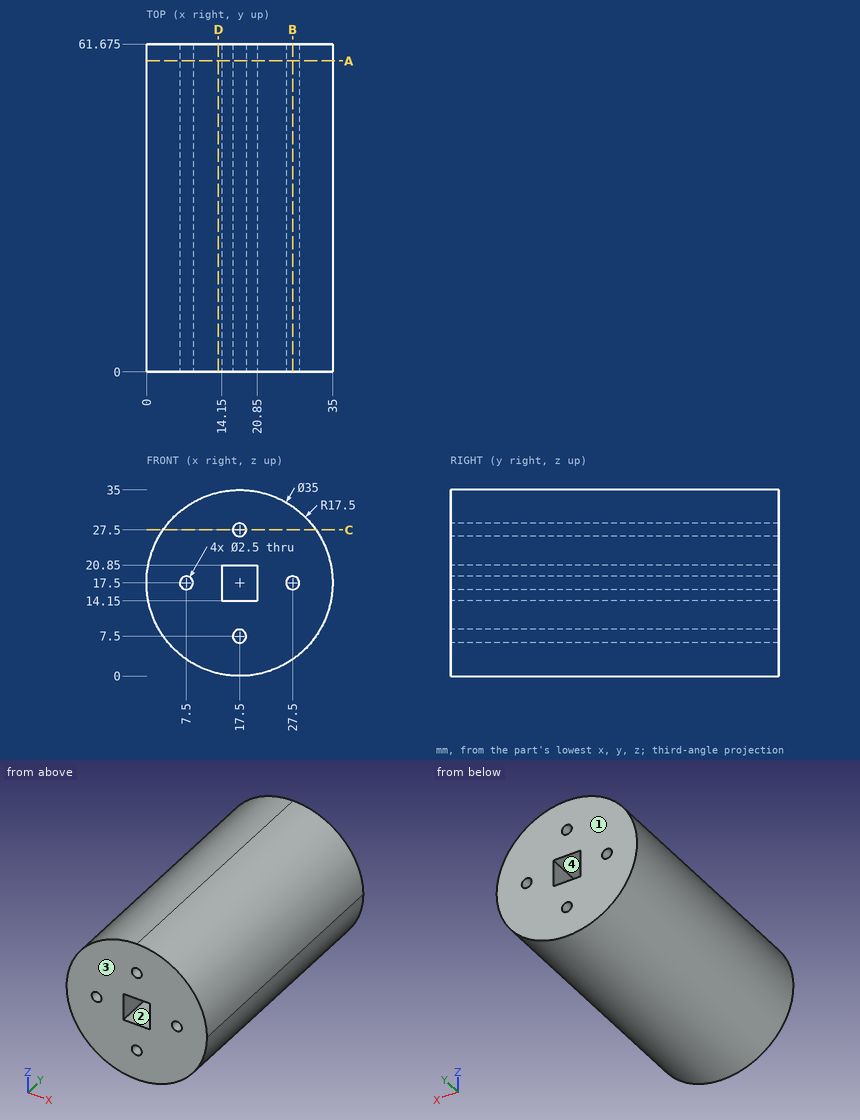
Drawing for the job (mm, zero at the part's lowest x, y, z). A direction names the side the tool comes from. Give positions to 0.01 mm unless a question says otherwise; leave off trailing zeros. Write each loop counter-clockwise with the first axis right and the second up, starting at its lowest first coordinate (ties: lowest second). Pieces come first, ordered by that corner, then holes. Notation, with made-up numbers: (-21, -31.5) - (-17, -31.5) arc R38 cw to (-17, 6.5) - close; hole circle Ø8 at (20, 49). An arc over 180 degrees is marked (long way). Answer as CSV lines item,"result".
Q1. Band-saw the part on D-D (x = 13.5). Give the cut face in (y, z) (3 decimals), and give its area (3 significant figures).
Result set:
outline,"(0, 0.463) - (61.675, 0.463) - (61.675, 34.537) - (0, 34.537) - close"
area,"2,100 mm²"
Q2. Drill centre lines: line 1 (Z direction, x = 8.5, y = 16); line 2 (X direction, y = 52, z = 14.5); line 3 (X direction, y = 19, z = 7.5). Where is each one in solid material? Low to high. Write a range as from..to.
Result set:
line 1,"2.49..16.75, 18.25..32.51"
line 2,"0.26..14.15, 20.85..34.74"
line 3,"3.14..16.25, 18.75..31.86"
Q3. Pull direction X, two halves, no side cores. Call the marked faces 1 and 2: released by +X, released by -X, zero draft, split by the parting line, or undercut.
Result set:
face 1,"zero draft"
face 2,"undercut"
Q4. Band-saw the part on B-B (x = 27.5). Give the cut face in (y, z) (3 decimals).
Result set:
outline,"(0, 3.139) - (61.675, 3.139) - (61.675, 16.25) - (0, 16.25) - close; (0, 18.75) - (61.675, 18.75) - (61.675, 31.861) - (0, 31.861) - close"
Q5. Flat gauge pins, fed straight in: pin 1 Ø1 at (x, y) = (21.5, 41) entering from -Z; pin 2 Ø12 at (x, y) = (4, 11) entering from -Z; pin 3 Ø5 at (x, y) = (29.5, 8) entering from -Z; pin 4 Ø2 at (x, z) = (17.5, 7.5) entering from -Y. Where does each tip first touch, or does it go through?
Result set:
pin 1,"z = 0.35"
pin 2,"z = 1.69"
pin 3,"z = 2.8"
pin 4,"through"
Q6. Band-saw the part on C-C (z = 27.5). Give the cut face in (x, y) (3 decimals).
Result set:
outline,"(3.139, 0) - (16.25, 0) - (16.25, 61.675) - (3.139, 61.675) - close; (18.75, 0) - (31.861, 0) - (31.861, 61.675) - (18.75, 61.675) - close"
Q7. 3-axis set-ups, long thin cutter, end or side, ignore diameter. For the marked faces 3 and 4: which of +Z, -Z, +X, -X, +Y, -Y reach the whole face in a straight line?
Result set:
face 3,"+Z, -Z, +X, -X, -Y"
face 4,"+Y, -Y"
Q8. Band-saw the part on A-A (y = 58.5). Give the cut face in (x, z).
Result set:
outline,"circle Ø35 at (17.5, 17.5); hole circle Ø2.5 at (7.5, 17.5); hole (14.15, 14.15) - (20.85, 14.15) - (20.85, 20.85) - (14.15, 20.85) - close; hole circle Ø2.5 at (17.5, 7.5); hole circle Ø2.5 at (17.5, 27.5); hole circle Ø2.5 at (27.5, 17.5)"
